Model file for the job. Use its own axes, mm. A direction names the side the tool comes from. Round coordinates to 2 decimals unless told otherwise and drop trailing zeros. Order: outer loops, then holes, each group sorted by start corner. A loop starts at its lowest first (then second) coordinate and runs counter-clockwise, first axis right, second up. Notation, with made-up numbers: (12, 19) - (53, 19) arc R20 cw to (53, 32) - close; hole circle Ø10 at (81.5, 87). An arc over 180 degrees is marked (long way). Write item = value, one per line.
```python
from build123d import *

# Parameters (mm, degrees)
ESBO_O1_W                = 40
ESBO_O1_H                = 40
ESBO_O1_R                = 2
ESBO_O1_R_2              = 1.75
ESBO_O1_R_3              = 11
RESSALTO_EXTRUS_O1_DEPTH = 6
CHANFRO1_SIZE            = 4
FILETE1_R                = 5


with BuildPart() as part:
    # Esboço1 → Ressalto-extrusão1 (new body)
    # profile 1 of 2: a face of its own
    with BuildSketch(Plane.XY):
        with Locations((20, 20)):
            Rectangle(ESBO_O1_W, ESBO_O1_H)
        with Locations((30, 30)):
            Circle(ESBO_O1_R, mode=Mode.SUBTRACT)
        with Locations((10, 10)):
            Circle(ESBO_O1_R, mode=Mode.SUBTRACT)
        with Locations((30, 10)):
            Circle(ESBO_O1_R, mode=Mode.SUBTRACT)
    # profile 2 of 2: a face of its own
    with BuildSketch(Plane.XY):
        Polygon((40, 40), (40, 9), (82, 9), (82, 51), (40, 51), align=None)
        with Locations((45.5, 14.5)):
            Circle(ESBO_O1_R_2, mode=Mode.SUBTRACT)
        with Locations((76.5, 14.5)):
            Circle(ESBO_O1_R_2, mode=Mode.SUBTRACT)
        with Locations((61, 30)):
            Circle(ESBO_O1_R_3, mode=Mode.SUBTRACT)
        with Locations((45.5, 45.5)):
            Circle(ESBO_O1_R_2, mode=Mode.SUBTRACT)
        with Locations((76.5, 45.5)):
            Circle(ESBO_O1_R_2, mode=Mode.SUBTRACT)
    extrude(amount=RESSALTO_EXTRUS_O1_DEPTH)

    # Chanfro1
    chanfro1_edges = [part.edges().sort_by_distance(p)[0] for p in [
        (40, 51, 3),
        (82, 51, 3),
        (82, 9, 3),
    ]]
    chamfer(chanfro1_edges, length=CHANFRO1_SIZE)

    # Filete1
    filete1_edges = [part.edges().sort_by_distance(p)[0] for p in [
        (40, 40, 3),
        (40, 9, 3),
    ]]
    fillet(filete1_edges, radius=FILETE1_R)


solid = part.part
```
1) 3-axis set-ups, long thin cutter, end or side, ignore diameter. For faces 1 (the face through (40, 46, 3)), 2 (the face through (61, 9, 3)), 3 (the face through (47.169, 15.026, 2.958)): which of +Z, -Z, +X, -X, +Y, -Y reach the whole face in a straight line?
Conclusion:
face_1 = +Z, -Z, -X, +Y
face_2 = +Z, -Z, +X, -Y
face_3 = +Z, -Z
2) Cut at D-D (z = 3). Give the number of separate pieces and of enclosed holes in the cut face, and give its area (3 significant figures).
Conclusion:
separate_pieces = 1
enclosed_holes = 8
area = 2,890 mm^2
3) Wall check: line 1 along Y through (x, z) = (45.5, 4.65); line 2 along Y through (x, z) = (30, 3.6); line 3 along Y through (x, z) = (10, 3.5). Give the ranges that are in metal, low to high.
Conclusion:
line_1 = 9 to 12.75, 16.25 to 43.75, 47.25 to 51
line_2 = 0 to 8, 12 to 28, 32 to 40
line_3 = 0 to 8, 12 to 40
4) Cut at B-B (x = 30). Write the cut outline in (y, z), and give its area (3 significant figures).
Conclusion:
outline = (0, 0) - (8, 0) - (8, 6) - (0, 6) - close; (12, 0) - (28, 0) - (28, 6) - (12, 6) - close; (32, 0) - (40, 0) - (40, 6) - (32, 6) - close
area = 192 mm^2
5) Cut at A-A (y = 14.5). Write the cut outline in (x, z).
Conclusion:
outline = (0, 0) - (43.75, 0) - (43.75, 6) - (0, 6) - close; (47.25, 0) - (74.75, 0) - (74.75, 6) - (47.25, 6) - close; (78.25, 0) - (82, 0) - (82, 6) - (78.25, 6) - close
6) Cut at C-C (x = 61). Write the cut outline in (y, z), and give its area (3 significant figures).
Conclusion:
outline = (9, 0) - (19, 0) - (19, 6) - (9, 6) - close; (41, 0) - (51, 0) - (51, 6) - (41, 6) - close
area = 120 mm^2
7) Mould opens along X. For faces 4 (the face through (42, 8, 3)), 5 (the face through (20, 0, 3)), 6 (the face through (30.923, 28.226, 2.958)), 7 (the face through (31.908, 10.601, 2.958)) say: +X half, -X half, draft (parallel to the pull), parting line (faces both ways), or undercut.
Conclusion:
face_4 = +X half
face_5 = draft
face_6 = undercut
face_7 = undercut
8) Flat gauge pins, fed straight in: pin 1 Ø3 at (x, y) = (76.5, 14.5) entering from -Z; pin 2 Ø0.6 at (y, z) = (46, 2.5) entering from -X; pin 3 Ø1 at (y, z) = (41.5, 2) entering from -X; pin 4 Ø2 at (y, z) = (2, 2) entering from +X. Where does each tip first touch, or does it go through?
Conclusion:
pin_1 = through
pin_2 = 40
pin_3 = 38
pin_4 = 40
